```python
from build123d import *

# Parameters (mm, degrees)
BOSS_EXTRUDE1_DEPTH  = 35
CONVERT_SOLID1_DEPTH = 35


# Read off the part's stored shape, not the designer's step: Convert-Solid1
with BuildPart() as part:
    # Sketch1 → Boss-Extrude1 (new body)
    with BuildSketch(Plane.XY):
        with BuildLine():
            Line((0, 0), (40, 0))
            ThreePointArc((40, 0), (44.770067359, 1.975826594), (46.745893953, 6.745893953))
            Line((46.745893953, 6.745893953), (46.745893953, 36.745893953))
            ThreePointArc((46.745893953, 36.745893953), (44.768864726, 41.518864726), (39.995893953, 43.495893953))
            Line((39.995893953, 43.495893953), (-0.004106047, 43.495893953))
            Line((-0.004106047, 43.495893953), (-0.004106047, 41.995893953))
            Line((-0.004106047, 41.995893953), (39.995893953, 41.995893953))
            ThreePointArc((39.995893953, 41.995893953), (43.708204554, 40.458204554), (45.245893953, 36.745893953))
            Line((45.245893953, 36.745893953), (45.245893953, 6.75))
            ThreePointArc((45.245893953, 6.75), (43.708204554, 3.037689399), (39.995893953, 1.5))
            Line((39.995893953, 1.5), (0, 1.5))
            Line((0, 1.5), (0, 0))
        make_face()
    extrude(amount=BOSS_EXTRUDE1_DEPTH)

    # Convert-Solid1 outline → Convert-Solid1 (add)
    with BuildSketch(Plane.XY):
        with BuildLine():
            Line((39.995893953, 41.995893953), (-0.004106047, 41.995893953))
            Line((-0.004106047, 41.995893953), (-0.004106047, 41.495893953))
            Line((-0.004106047, 41.495893953), (39.995893953, 41.495893953))
            ThreePointArc((39.995893953, 41.495893953), (43.354651163, 40.104651163), (44.745893953, 36.745893953))
            Line((44.745893953, 36.745893953), (44.745893953, 6.745893953))
            ThreePointArc((44.745893953, 6.745893953), (43.355853797, 3.390040156), (40, 2))
            Line((40, 2), (0, 2))
            Line((0, 2), (0, 1.5))
            Line((0, 1.5), (39.995893953, 1.5))
            ThreePointArc((39.995893953, 1.5), (43.708204554, 3.037689399), (45.245893953, 6.75))
            Line((45.245893953, 6.75), (45.245893953, 36.745893953))
            ThreePointArc((45.245893953, 36.745893953), (43.708204554, 40.458204554), (39.995893953, 41.995893953))
        make_face()
    extrude(amount=CONVERT_SOLID1_DEPTH)


solid = part.part
```
Source: CAD feature listing. Evaluate the final solid. Frame: model axes, mm. A direction names the side the tool comes from. Coordinates: 2 decimals unless noted, no trailing zeros. Loops run counter-clockwise (first coordinate to the right, second up) from the corner with the lowest first, then second, coordinate; pieces in that order, holes last. Notation, with made-up numbers: (79.25, 6) -> (94.25, 6) arc R22 cw to (94.25, 17) -> close; hole circle Ø6 at (-21.5, 29). An arc over 180 degrees is marked (long way). One line per item, written item: value. Start each with the question number.
Q1. Section query D-D, the plane y = 6. Return the cut outline in (x, z), and give its area (3 significant figures).
Q2. Section query A-A, the plane x = 31. Return the cut outline in (y, z), and give its area (3 significant figures).
Q3. Section query B-B, the plane z = 23. Return the cut outline in (x, y).
Q4. Mould query, pull axis Y, two halves, no side actions, for faces 3 (the face through (44.746, 22, 17)), 4 (the face through (20, 0, 17)), 5 (the face through (46, 22, 35)). Classes: pulls with the +Y half, pulls with the -Y half, needs draft (parallel to the pull), parting line crosses it, or undercut.
Q5. Section query C-C, the plane y = 33. Return the cut outline in (x, z), and give its area (3 significant figures).
Q6. Set-up query: faces 1 (the face through (20, 43.496, 17)), 2 (the face through (43.32, 40.14, 17.26)). Return all of +Z, -Z, +X, -X, +Y, -Y with unobstructed straight access to the full face (end or side cutting, diameter ignored); none if empty.
Q7. Contact query for flat-ended pins moving along their axis: P1, Ø4, axis at x = 33.5, y = 38.5, coming from the +Z side; P2, Ø1, axis at y = 1, z = 20.5, coming from the -X side. Output: stop coordinate, or through.
Q8. Line query: line 1 along Y through (x, z) = (34, 32.5); line 2 along X through (y, z) = (32, 4); line 3 along Y through (x, z) = (41, 19). Output: solid intervals per line, ascending.
Results:
1. outline: (44.69, 0) -> (46.7, 0) -> (46.7, 35) -> (44.69, 35) -> close
1. area: 70.6 mm^2
2. outline: (0, 0) -> (2, 0) -> (2, 35) -> (0, 35) -> close; (41.5, 0) -> (43.5, 0) -> (43.5, 35) -> (41.5, 35) -> close
2. area: 140 mm^2
3. outline: (0, 0) -> (40, 0) arc R6.75 ccw to (46.75, 6.75) -> (46.75, 36.75) arc R6.75 ccw to (40, 43.5) -> (0, 43.5) -> (0, 41.5) -> (40, 41.5) arc R4.75 cw to (44.75, 36.75) -> (44.75, 6.75) arc R4.75 cw to (40, 2) -> (0, 2) -> close
4. face 3: undercut
4. face 4: pulls with the -Y half
4. face 5: needs draft
5. outline: (44.75, 0) -> (46.75, 0) -> (46.75, 35) -> (44.75, 35) -> close
5. area: 70.0 mm^2
6. face 1: +Z, -Z, +X, -X, +Y
6. face 2: +Z, -Z, -X
7. P1: through
7. P2: x = 0
8. line 1: 0 to 2, 41.5 to 43.5
8. line 2: 44.75 to 46.75
8. line 3: 0.07 to 2.11, 41.39 to 43.42
